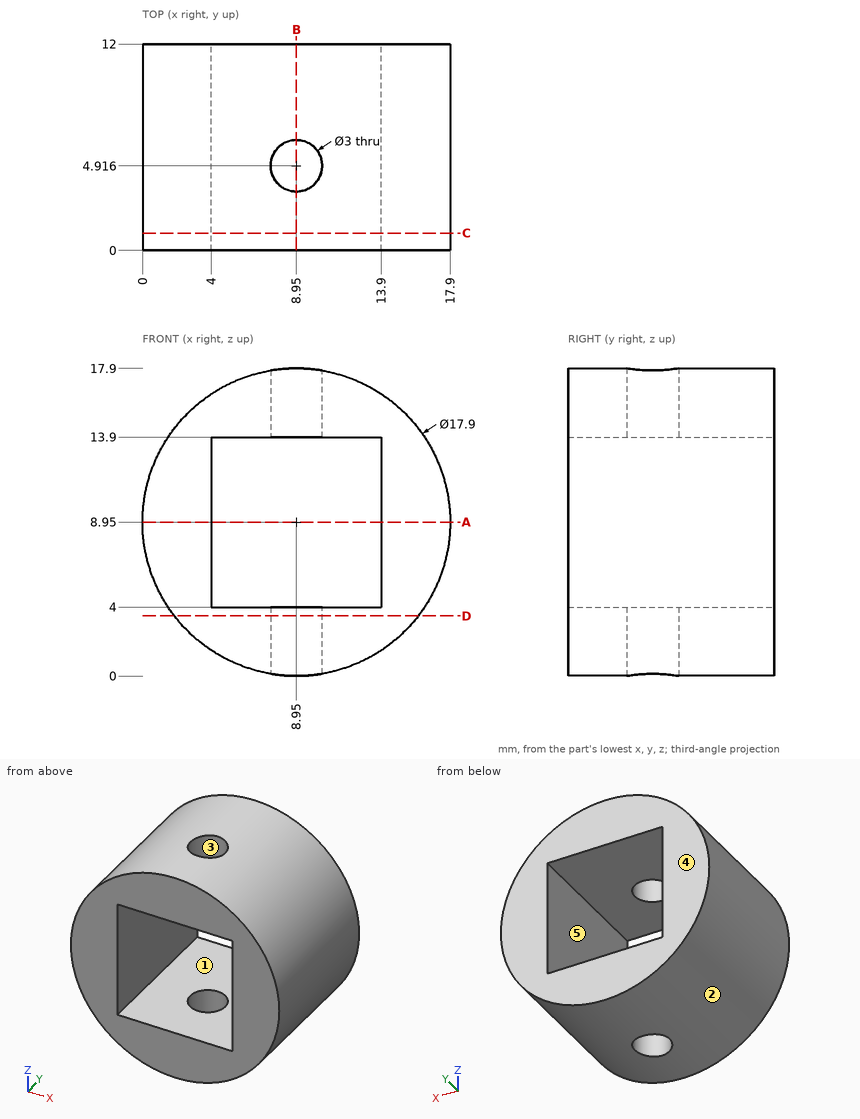
Verification items for this drawing (mm, ordinates from the low corner). A direction names the side the tool comes from. Coordinates: 2 decimals unless noted, no trailing zeros. Write each loop counter-clockwise with the first axis right and the second up, starting at its lowest first coordinate (ties: lowest second). Pieces come first, ordered by that corner, then holes. Notation, with made-up numbers: M -18.5,-16 L 0.5,-16 A19 ccw 0.5,2 Z; hole C 36,-33.75 d7. An arc over 180 degrees is marked long. Use CSV: the item, a comma, the result in double quotes.
Q1. Section check C-C, the plane y = 1. Enter the section's corners in (x, z), and give its area (3 significant figures).
Computed values:
outline,"C 8.95,8.95 d17.9; hole M 4,4 L 13.9,4 L 13.9,13.9 L 4,13.9 Z"
area,"154 mm²"
Q2. Mould release check, pull along Z, two halves, no side actions. Record for the marked faces 1, 2 and 3: pulls with the +Z half, pulls with the -Z half, needs draft (parallel to the pull), parting line crosses it, or undercut.
Computed values:
face 1,"undercut"
face 2,"parting line crosses it"
face 3,"needs draft"
Q3. Go/stop test with flat-tipped pins: P1, Ø1, axis at x = 3, y = 7.5, coming from the +Z side; P2, Ø2.5, axis at x = 8.95, y = 4.92, coming from the -Z side; P3, Ø5, axis at y = 5, z = 3.5, coming from the -X side; P4, Ø1, axis at x = 15.5, y = 3, coming from the +Z side (1 decimal). Record where each tip stops, or that it passes through.
Computed values:
P1,"z = 16.05"
P2,"through"
P3,"x = 0.5"
P4,"z = 15.5"
Q4. Set-up check for the marked faces 4 and 5: record each of +Z, -Z, +X, -X, +Y, -Y from which the full face is reachable in a straight line by a thin tool's end or side.
Computed values:
face 4,"+Z, -Z, +X, -X, +Y"
face 5,"+Y, -Y"
Q5. Section check B-B, the plane x = 8.95. Enter the section's corners in (y, z).
Computed values:
outline,"M 0,0 L 3.42,0 L 3.42,4 L 0,4 Z; M 0,13.9 L 3.42,13.9 L 3.42,17.9 L 0,17.9 Z; M 6.42,0 L 12,0 L 12,4 L 6.42,4 Z; M 6.42,13.9 L 12,13.9 L 12,17.9 L 6.42,17.9 Z"
Q6. Section check A-A, the plane z = 8.95. Enter the section's corners in (x, y).
Computed values:
outline,"M 0,0 L 4,0 L 4,12 L 0,12 Z; M 13.9,0 L 17.9,0 L 17.9,12 L 13.9,12 Z"
Q7. Thickness scan on line 1 along Z through (x, y) = (8.75, 11); line 2 along Y through (x, z) = (8.95, 15.1); line 3 along Z through (x, y) = (6.75, 2) (1 decimal). Record the ranges inside material, lowest first. Write a range as [from, to].
Computed values:
line 1,"[0, 4], [13.9, 17.9]"
line 2,"[0, 3.42], [6.42, 12]"
line 3,"[0.3, 4], [13.9, 17.6]"
Q8. Section check D-D, the plane z = 3.5. Enter the section's corners in (x, y), and give its area (3 significant figures).
Computed values:
outline,"M 1.85,0 L 16.05,0 L 16.05,12 L 1.85,12 Z; hole C 8.95,4.92 d3"
area,"163 mm²"
